Input: part model. Units: mm. Frame: model coordinates. Face numbers are marked on the shaded views. Coordinates: 2 decimals unless noted, no trailing zeros. Loops run counter-clockwise (first coordinate to the right, second up) from the corner with the lowest first, then second, coordinate; pieces in that order, holes last. Notation, with made-up numbers: (66.25, -22.75) -> (109.25, -22.75) arc R31 ccw to (109.25, 8.25) -> close; hole circle Ø5 at (8, 39). An arc over 180 degrees is marked (long way). Put each result on its own line as item: value. Start each with the question number.
1) Cut plane B-B (y = -10). Return the cut outline in (x, z).
2) Cut plane C-C (z = 1.95). Return the cut outline in (x, y), plus the area to 3 significant figures.
3) Cut plane D-D (y = -1.5). Return the cut outline in (x, z).
4) Cut plane A-A (x = -10.5). Return the cut outline in (y, z).
5) Pull-direction query (Y, two-part tool) for the marked faces 1, 2 and 3; classes: pulls with the +Y half, pulls with the -Y half, needs draft (parallel to the pull), parting line crosses it, or undercut.
6) Material intervals for L1, parallel to Y at x = 10.5, z = 2.3; L2, parallel to Y at x = -15, z = 3.7; L3, parallel to X at y = -2, z = 1.35, sorted ascending.
7) Contact query for flat-ended pins moving along their axis: P1, Ø1.7, axis at x = 10.5, y = -10, coming from the +Z side; P2, Ø1, axis at y = 12.5, z = 1, coming from the +X side; P3, Ø2, axis at y = 3.5, z = 3.5, coming from the +X side. Output: stop coordinate, or through.
from build123d import *

# Parameters (mm, degrees)
SKETCH1_W           = 40
SKETCH1_H           = 33.426210179
BOSS_EXTRUDE1_DEPTH = 4
SKETCH2_R           = 1.05
CUT_EXTRUDE1_DEPTH  = 28.486819051
SKETCH3_R           = 9
CUT_EXTRUDE2_DEPTH  = 5


with BuildPart() as part:
    # Sketch1 → Boss-Extrude1 (new body)
    with BuildSketch(Plane.XY):
        with Locations((0, 1.713105089)):
            Rectangle(SKETCH1_W, SKETCH1_H)
    extrude(amount=BOSS_EXTRUDE1_DEPTH)

    # Sketch2 → Cut-Extrude1 (cut, through all)
    with BuildSketch(Plane(origin=(0, 0, 0), x_dir=(-1, 0, 0), z_dir=(0, 0, -1))):
        with Locations((-10.5, 2.5)):
            Circle(SKETCH2_R)
        with Locations((10.5, 2.5)):
            Circle(SKETCH2_R)
        with Locations((-10.5, -10)):
            Circle(SKETCH2_R)
        with Locations((10.5, -10)):
            Circle(SKETCH2_R)
    extrude(amount=-CUT_EXTRUDE1_DEPTH, mode=Mode.SUBTRACT)

    # Sketch3 → Cut-Extrude2 (cut)
    with BuildSketch(Plane.XY.offset(4)):
        with Locations((22, 5.687428233)):
            Circle(SKETCH3_R)
        with Locations((-22, 5.687428233)):
            Circle(SKETCH3_R)
    extrude(amount=-CUT_EXTRUDE2_DEPTH, mode=Mode.SUBTRACT)


solid = part.part
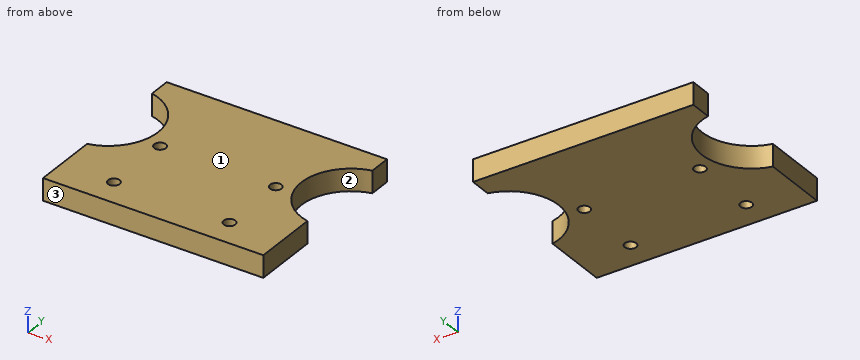
Results found:
1. outline: (-20, 0) -> (-11.55, 0) -> (-11.55, 4) -> (-20, 4) -> close; (-9.45, 0) -> (9.45, 0) -> (9.45, 4) -> (-9.45, 4) -> close; (11.55, 0) -> (20, 0) -> (20, 4) -> (11.55, 4) -> close
2. outline: (-20, -15) -> (20, -15) -> (20, -3.09) arc R9 cw to (20, 14.46) -> (20, 18.43) -> (-20, 18.43) -> (-20, 14.46) arc R9 cw to (-20, -3.09) -> close; hole circle Ø2.1 at (-10.5, -10); hole circle Ø2.1 at (-10.5, 2.5); hole circle Ø2.1 at (10.5, -10); hole circle Ø2.1 at (10.5, 2.5)
2. area: 1,140 mm2
3. outline: (-16.58, 0) -> (16.58, 0) -> (16.58, 4) -> (-16.58, 4) -> close
4. outline: (-15, 0) -> (-11.05, 0) -> (-11.05, 4) -> (-15, 4) -> close; (-8.95, 0) -> (1.45, 0) -> (1.45, 4) -> (-8.95, 4) -> close; (3.55, 0) -> (18.43, 0) -> (18.43, 4) -> (3.55, 4) -> close
5. face 1: needs draft
5. face 2: undercut
5. face 3: pulls with the -Y half
6. L1: y = -15 to -11.05, -8.95 to 1.45, 3.55 to 18.43
6. L2: y = -15 to 0.03, 11.34 to 18.43
6. L3: x = -17.32 to 17.32
7. P1: passes through
7. P2: stops at x = 16.75
7. P3: stops at x = 13.58
